Here's the drawing with two shaded views (mm, measured from the low corner). I have some questions. A direction names the side the tool comes from. Give positions to 0.01 mm unless a question says otherwise; leave off trailing zeros. Write each loop counter-clockwise with the first axis right and the second up, starting at its lowest first coordinate (ties: lowest second). Pieces come first, ordered by that corner, then holes. Notation, with made-up numbers: (-23.5, -22.75) -> (-19.5, -22.75) arc R13 cw to (-19.5, -15.75) -> close; hole circle Ø9 at (-21.5, 9.5). An arc over 180 degrees is marked (long way). One line per item, written item: value.
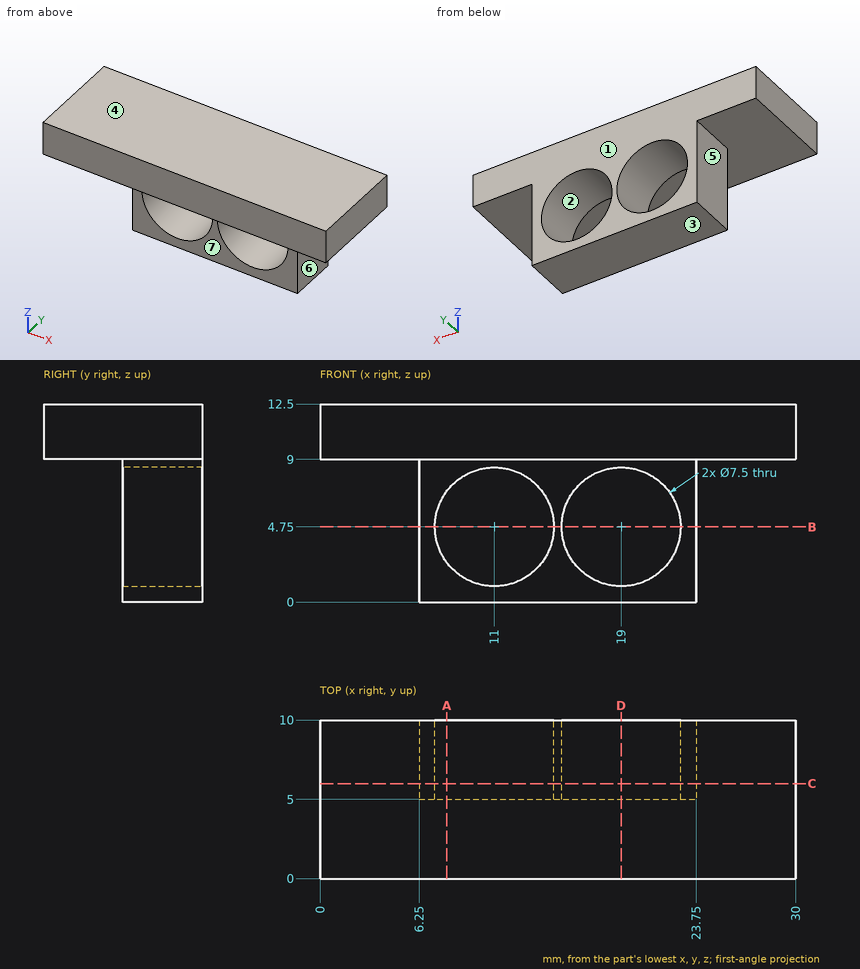
1) If we section it at D-D (x = 19): Write out the boundary of the cut face in (y, z), and give its area (3 significant figures).
Answer list:
outline: (0, 9) -> (5, 9) -> (5, 8.5) -> (10, 8.5) -> (10, 12.5) -> (0, 12.5) -> close; (5, 0) -> (10, 0) -> (10, 1) -> (5, 1) -> close
area: 42.5 mm^2
2) We'd pull the mould along Z, two halves only. Please class the marked faces 1, 2, 3 and 4: released by +Z, released by -Z, zero draft, split by the parting line, or undercut.
Answer list:
face 1: zero draft
face 2: undercut
face 3: released by -Z
face 4: released by +Z
3) If we section it at C-C (y = 6): Write out the boundary of the cut face in (x, z).
Answer list:
outline: (0, 9) -> (6.25, 9) -> (6.25, 0) -> (23.75, 0) -> (23.75, 9) -> (30, 9) -> (30, 12.5) -> (0, 12.5) -> close; hole circle Ø7.5 at (11, 4.75); hole circle Ø7.5 at (19, 4.75)
4) For the marked faces 5, 6 and 7, which set-ups out of +Z, -Z, +X, -X, +Y, -Y let a thin tool reach every point of the face, with its end or its side?
Answer list:
face 5: -Z, -X, +Y, -Y
face 6: -Z, +X, +Y, -Y
face 7: -Z, +X, -X, -Y
5) I need wall thicknesses on L1, parallel to X at y = 6.9, z = 4.75; L2, parallel to X at y = 9.75, z = 7; L3, parallel to Z at x = 15.5, y = 4. Which ranges of each line are inside material? Lowest first, please.
Answer list:
L1: x = 6.25 to 7.25, 14.75 to 15.25, 22.75 to 23.75
L2: x = 6.25 to 8, 14 to 16, 22 to 23.75
L3: z = 9 to 12.5
6) If we section it at B-B (z = 4.75): Write out the boundary of the cut face in (x, y).
Answer list:
outline: (6.25, 5) -> (7.25, 5) -> (7.25, 10) -> (6.25, 10) -> close; (14.75, 5) -> (15.25, 5) -> (15.25, 10) -> (14.75, 10) -> close; (22.75, 5) -> (23.75, 5) -> (23.75, 10) -> (22.75, 10) -> close
7) Will these pins go through, and if not, where does the flat tip stop? pin 1 (6 mm diameter, centred on x = 11, z = 4.75, fed in from +Y); pin 2 (4 mm diameter, centred on y = 7, z = 5, fed in from -X); pin 3 (4.5 mm diameter, centred on x = 14.5, z = 5.5, fed in from -Y); pin 4 (4 mm diameter, centred on x = 5, y = 2, fed in from -Z).
Answer list:
pin 1: passes through
pin 2: stops at x = 6.25
pin 3: stops at y = 5
pin 4: stops at z = 9
8) If we section it at A-A (x = 8): Write out the boundary of the cut face in (y, z).
Answer list:
outline: (0, 9) -> (5, 9) -> (5, 7) -> (10, 7) -> (10, 12.5) -> (0, 12.5) -> close; (5, 0) -> (10, 0) -> (10, 2.5) -> (5, 2.5) -> close
